Design review of the part built by this model. Coordinates are the model's own, in mm. Face numbers are marked on the shaded views. A direction names the side the tool comes from. Coordinates: 2 decimals unless noted, no trailing zeros. Loops run counter-clockwise (first coordinate to the right, second up) from the corner with the lowest first, then second, coordinate; pieces in that order, holes last. Notation, with made-up numbers: (-37.5, -32.75) -> (-8.5, -32.75) arc R33 ccw to (-8.5, 4.25) -> close; hole circle Ø3 at (-1, 14). An arc over 180 degrees is marked (long way). Use a Markdown table: item, result. Add a question column.
Q1. For probe 1 along Z at (x, y) = (16, -2); probe 2 along Z at (x, y) = (-1.5, -6); probe 3 along X at (y, z) = (-2.25, 5.5), list the stretches that pass through material, from the lowest coordinate up.
Q2. Draft analysis for pull direction X (two halves, no side actions). For the marked faces 1, 2, 3 and 4, state which applies: pulls with the +X half, pulls with the -X half, needs draft (parallel to the pull), parting line crosses it, or undercut.
Q3. Take a section at A-A on x = 12. Write out the cut boundary in (y, z), plus the area to 3 significant figures.
Q4. Clearance check with a flat-ended pin moving along its axis: pin 1 Ø1 at (y, z) = (-1.5, -5) entering from +X. State where the tip first meets the part, or that it passes through.
Q5. For the marked faces 5 and 6, list the 3-axis set-ups (+Z, -Z, +X, -X, +Y, -Y) from which the entire face can be reached by the end or side of a thin tool; tool diameter is ignored.
Q6. Take a section at B-B on y = -1.25. Write out the cut boundary in (x, z).
Q7. Take a section at D-D on z = -8.5. Write out the cut boundary in (x, y), plus the area to 3 significant figures.
Q8. Take a section at C-C on x = -7.5. Write out the cut boundary in (y, z).
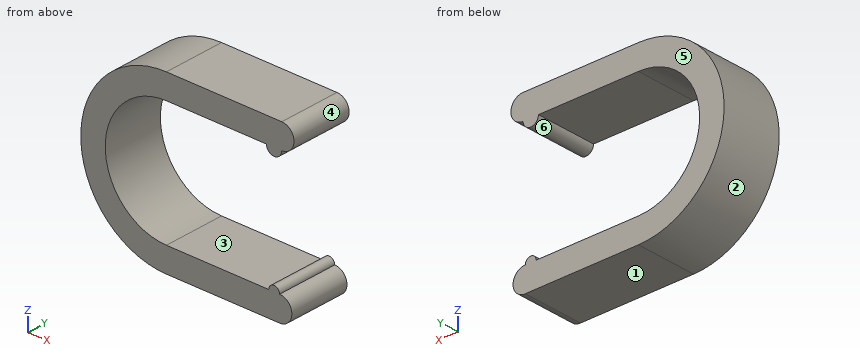
from build123d import *

# Parameters (mm, degrees)
F1_DEPTH = 10


with BuildPart() as f1:
    # F0 (on Front) → F1 (new body)
    with BuildSketch(Plane.XZ):
        with BuildLine():
            ThreePointArc((0, -10), (-10, 0), (0, 10))
            Line((0, 10), (16.356886, 10))
            Line((16.356886, 10), (18.862135, 10))
            Line((18.862135, 10), (18.862135, 14))
            Line((18.862135, 14), (0, 14))
            ThreePointArc((0, 14), (-14, 0), (0, -14))
            Line((0, -14), (18.509572, -14))
            Line((18.509572, -14), (18.509572, -10))
            Line((18.509572, -10), (16.730837, -10))
            Line((16.730837, -10), (0, -10))
        make_face()
        with BuildLine():
            Line((18.862135, 14), (18.862135, 10))
            ThreePointArc((18.862135, 10), (20.862135, 12), (18.862135, 14))
        make_face()
        with BuildLine():
            Line((18.862135, 10), (16.356886, 10))
            ThreePointArc((16.356886, 10), (17.60951, 8.747376), (18.862135, 10))
        make_face()
        with BuildLine():
            ThreePointArc((18.509572, -14), (20.509572, -12), (18.509572, -10))
            Line((18.509572, -10), (18.509572, -14))
        make_face()
        with BuildLine():
            ThreePointArc((18.509572, -10), (17.620205, -9.110632), (16.730837, -10))
            Line((16.730837, -10), (18.509572, -10))
        make_face()
    extrude(amount=F1_DEPTH)


solid = f1.part
Answer list:
| question | item | result |
|---|---|---|
| 1 | probe 1 | -14 to -10, 10 to 14 |
| 1 | probe 2 | -13.92 to -9.89, 9.89 to 13.92 |
| 1 | probe 3 | -12.87 to -8.35 |
| 2 | face 1 | needs draft |
| 2 | face 2 | pulls with the -X half |
| 2 | face 3 | undercut |
| 2 | face 4 | pulls with the +X half |
| 3 | outline | (-10, -14) -> (0, -14) -> (0, -10) -> (-10, -10) -> close; (-10, 10) -> (0, 10) -> (0, 14) -> (-10, 14) -> close |
| 3 | area | 80.0 mm² |
| 4 | pin 1 | x = -8.35 |
| 5 | face 5 | +Z, -Z, +X, -X, +Y |
| 5 | face 6 | +Y, -Y |
| 6 | outline | (0, -14) -> (18.51, -14) arc R2 ccw to (18.51, -10) arc R0.89 ccw to (16.73, -10) -> (0, -10) arc R10 cw to (0, 10) -> (16.36, 10) arc R1.25 ccw to (18.86, 10) arc R2 ccw to (18.86, 14) -> (0, 14) arc R14 ccw to start |
| 7 | outline | (-11.12, -10) -> (-5.27, -10) -> (-5.27, 0) -> (-11.12, 0) -> close |
| 7 | area | 58.6 mm² |
| 8 | outline | (-10, -11.82) -> (0, -11.82) -> (0, -6.61) -> (-10, -6.61) -> close; (-10, 6.61) -> (0, 6.61) -> (0, 11.82) -> (-10, 11.82) -> close |
